Geometry check sheet. Reference: the model listing, model coordinates, mm. Coordinates: 2 decimals unless noted, no trailing zeros. Write each loop counter-clockwise with the first axis right and the second up, starting at its lowest first coordinate (ties: lowest second). Pieces come first, ordered by that corner, then holes. Notation, with made-up numbers: (0.25, -31.75) -> (57.25, -31.75) arc R18 cw to (57.25, -13.75) -> close; hole circle Ø5 at (61.5, 45). An arc over 180 degrees is marked (long way). Answer in a Markdown table with one row per item. Add a question column.
1. Cross-section at A-A on x = -347. Record the cut outline in (y, z), and give its area (3 significant figures).
2. Cross-section at B-B on y = -16.75. Record the cut outline in (x, z), and give its area (3 significant figures).
3. Depth check by flat-ended pin: P1, Ø4, axis at y = -24.5, z = 55, coming from the +X side; P2, Ø1, axis at y = -18, z = 41, coming from the -X side. Enter the tip coordinate at first touch or a pass-through.
4. Scan lines: L1, parallel to Z at x = 213, y = -23; L2, parallel to X at y = -25.5, z = 46; L3, parallel to Y at x = -204, z = 53. Record each from-to range of solid material in increasing order. Write a range as from..to.
5. Cross-section at C-C on z = 14. Record the cut outline in (x, y), and give its area (3 significant figures).
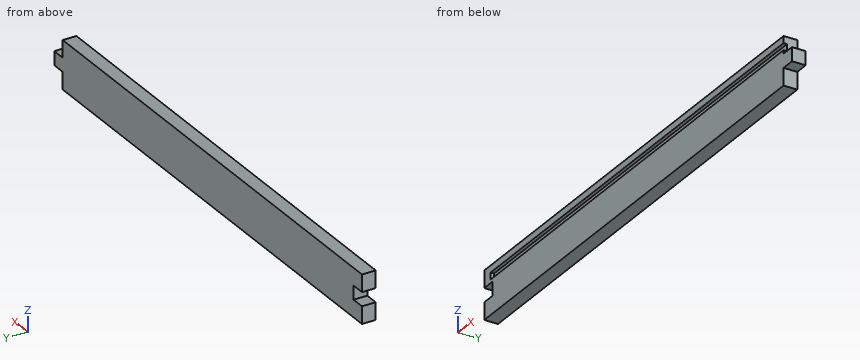
```python
from build123d import *

# Parameters (mm, degrees)
F0_W          = 730
F0_H          = 20
F1_DEPTH      = 70
F2_W          = 5
F2_H          = 10
F3_DEPTH      = 715
F3_DEPTH_BACK = 15
F4_W          = 20
F4_H          = 25
F4_H_2        = 20
F5_DEPTH      = 20.001


with BuildPart() as f1:
    # F0 (on Top) → F1 (new body)
    with BuildSketch(Plane.XY):
        with Locations((-39.742246, -17.948127)):
            Rectangle(F0_W, F0_H)
    extrude(amount=F1_DEPTH)

    # F2 (on face) → F3 (cut, two sides)
    with BuildSketch(Plane.YZ.offset(325.257754)) as f3_sk:
        with Locations((-25.448127, 55)):
            Rectangle(F2_W, F2_H)
    extrude(amount=-F3_DEPTH, mode=Mode.SUBTRACT)
    extrude(f3_sk.sketch, amount=-F3_DEPTH_BACK, mode=Mode.SUBTRACT)

    # F4 (on face) → F5 (cut, through all)
    with BuildSketch(Plane(origin=(0, -7.948127, 0), x_dir=(-1, 0, 0), z_dir=(0, 1, 0))):
        with Locations((-315.257754, 57.5)):
            Rectangle(F4_W, F4_H)
        with Locations((-315.257754, 12.5)):
            Rectangle(F4_W, F4_H)
        with Locations((394.742246, 35)):
            Rectangle(F4_W, F4_H_2)
    extrude(amount=-F5_DEPTH, mode=Mode.SUBTRACT)


solid = f1.part
```
Results found:
| question | item | result |
|---|---|---|
| 1 | outline | (-27.95, 0) -> (-7.95, 0) -> (-7.95, 70) -> (-27.95, 70) -> (-27.95, 60) -> (-22.95, 60) -> (-22.95, 50) -> (-27.95, 50) -> close |
| 1 | area | 1,350 mm^2 |
| 2 | outline | (-404.74, 0) -> (305.26, 0) -> (305.26, 25) -> (325.26, 25) -> (325.26, 45) -> (305.26, 45) -> (305.26, 70) -> (-404.74, 70) -> (-404.74, 45) -> (-384.74, 45) -> (-384.74, 25) -> (-404.74, 25) -> close |
| 2 | area | 49,700 mm^2 |
| 3 | P1 | stops at x = 305.26 |
| 3 | P2 | stops at x = -384.74 |
| 4 | L1 | z = 0..50, 60..70 |
| 4 | L2 | x = -404.74..305.26 |
| 4 | L3 | y = -22.95..-7.95 |
| 5 | outline | (-404.74, -27.95) -> (305.26, -27.95) -> (305.26, -7.95) -> (-404.74, -7.95) -> close |
| 5 | area | 14,200 mm^2 |
